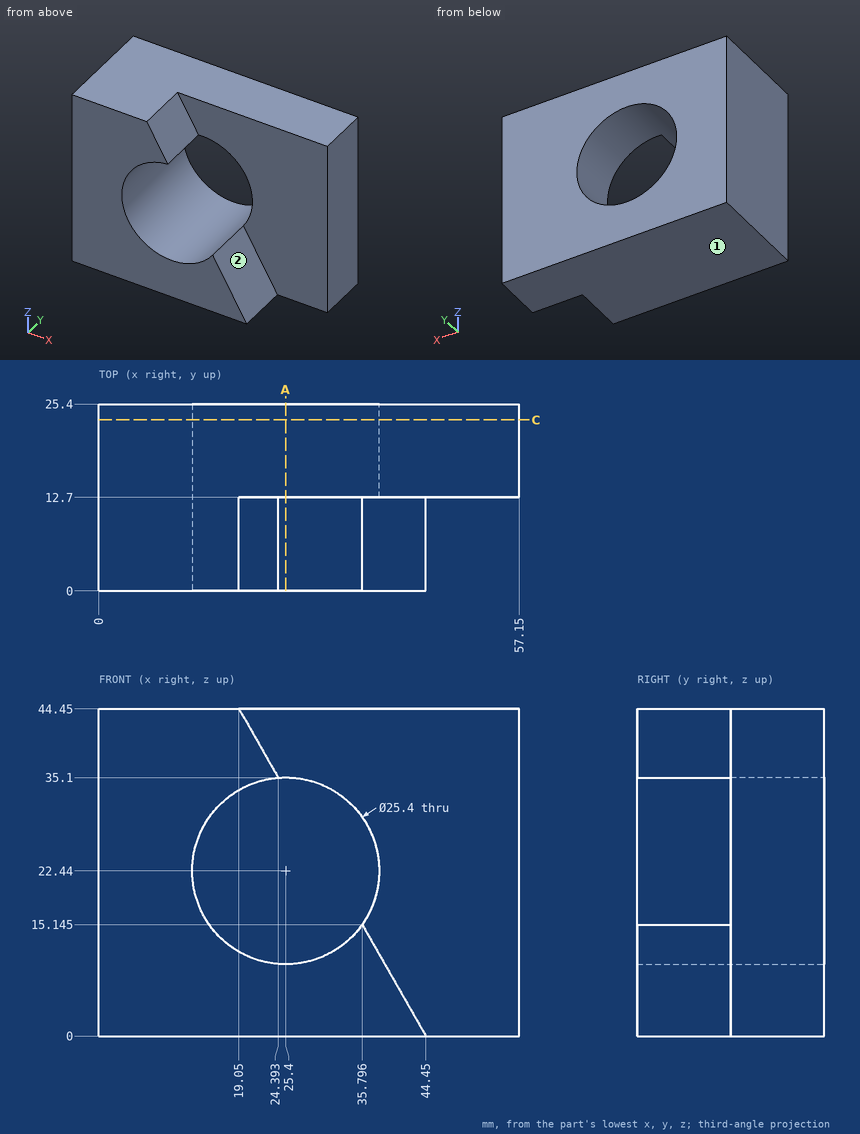
For this review, use the dimensioned drawing (mm, ordinates from the lowest corner) and the shaded views. A direction names the side the tool comes from. Coordinates: 2 decimals unless noted, no trailing zeros. Loops run counter-clockwise (first coordinate to the right, second up) from the corner with the lowest first, then second, coordinate; pieces in that order, holes last.
1. For the marked faces 1 and 2, list the 3-axis set-ups (+Z, -Z, +X, -X, +Y, -Y) from which the entire face can be reached by the end or side of a thin tool; tool diameter is ignored.
2. Add section A-A, the plane x = 25.4. Give the boundary of the cut face in (y, z), then the cut area to 3 significant figures.
3. For line 1 (Z direction, x = 25.4, y = 14.25); line 2 (Z direction, x = 25.4, y = 7); line 3 (Z direction, x = 27, y = 12.75), list the stretches that pass through material, from the lowest coordinate up.
4. Add section C-C, the plane y = 23.25. Give the boundary of the cut face in (x, z), then the cut area to 3 significant figures.
5. Insertion check: P1, Ø2, axis at x = 15.5, z = 20.5, coming from the +Y side. The pin has a flat end and moves straight along its axis. Give the tip position at first contact, or say it passes through.
Result:
1. face 1: -Z, +X, -X, +Y, -Y
1. face 2: +Z, +X, -Y
2. outline: (0, 0) - (25.4, 0) - (25.4, 9.74) - (0, 9.74) - close; (12.7, 35.14) - (25.4, 35.14) - (25.4, 44.45) - (12.7, 44.45) - close
2. area: 366 mm2
3. line 1: z = 0 to 9.74, 35.14 to 44.45
3. line 2: z = 0 to 9.74
3. line 3: z = 0 to 9.84, 35.04 to 44.45
4. outline: (0, 0) - (57.15, 0) - (57.15, 44.45) - (0, 44.45) - close; hole circle Ø25.4 at (25.4, 22.44)
4. area: 2,030 mm2
5. P1: passes through
